Drawing for the job (mm, zero at the part's lowest x, y, z). Coordinates: 2 decimals unless noted, no trailing zeros. Loops run counter-clockwise (first coordinate to the right, second up) from the corner with the lowest first, then second, coordinate; pieces in that order, holes last. Notation, with made-up numbers: (-1, 36) - (8, 36) arc R7 ccw to (8, 46) - close; hole circle Ø2 at (88.5, 88). An arc over 180 degrees is marked (long way). Put each result on its own line as item: value.
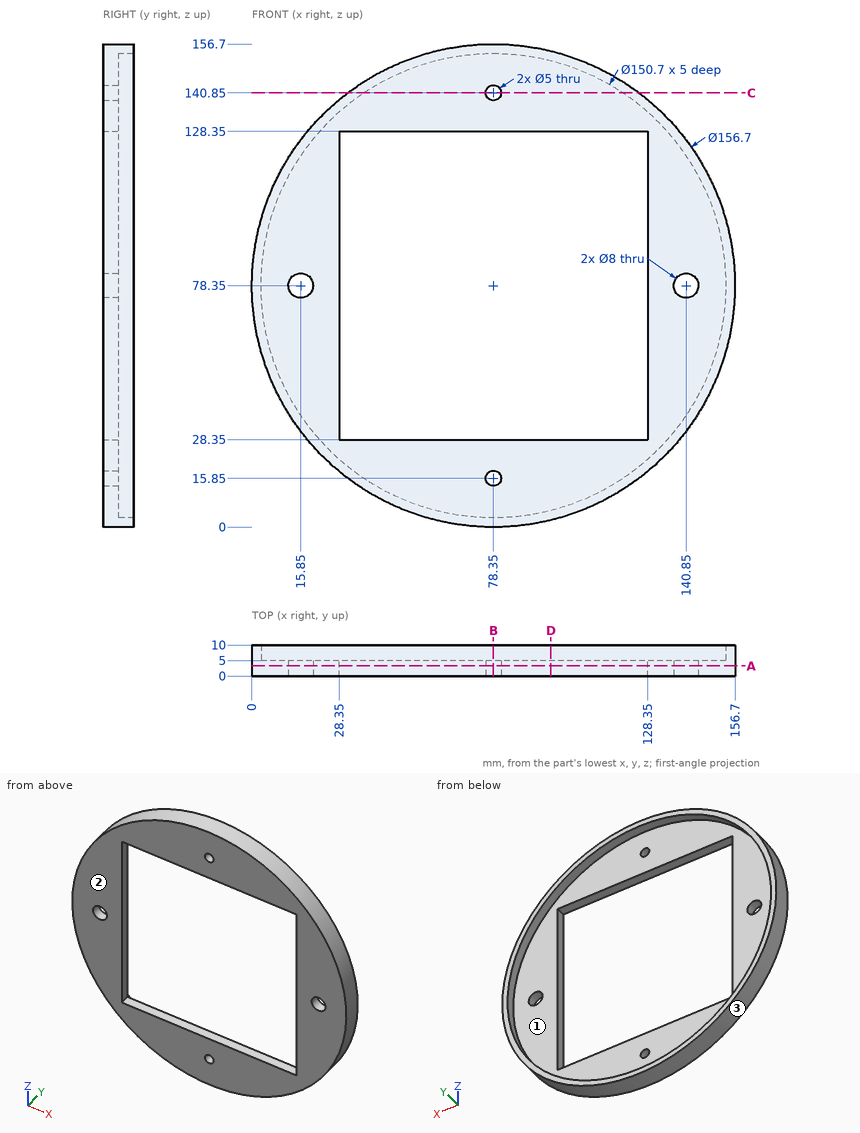
Q1. Slice it at D-D, the plane x = 97. Give the cut face in (y, z), then the cut area to 3 significant figures.
Determined:
outline: (0, 2.25) - (10, 2.25) - (10, 5.34) - (5, 5.34) - (5, 28.35) - (0, 28.35) - close; (0, 128.35) - (5, 128.35) - (5, 151.36) - (10, 151.36) - (10, 154.45) - (0, 154.45) - close
area: 292 mm2
Q2. Slice it at A-A, the plane y = 3.25. Give the cut face in (x, z).
Determined:
outline: circle Ø156.7 at (78.35, 78.35); hole circle Ø8 at (15.85, 78.35); hole (28.35, 28.35) - (128.35, 28.35) - (128.35, 128.35) - (28.35, 128.35) - close; hole circle Ø5 at (78.35, 15.85); hole circle Ø5 at (78.35, 140.85); hole circle Ø8 at (140.85, 78.35)
Q3. Slice it at B-B, the plane x = 78.35. Give the cut face in (y, z), then the cut area to 4 significant figures.
Determined:
outline: (0, 0) - (10, 0) - (10, 3) - (5, 3) - (5, 13.35) - (0, 13.35) - close; (0, 18.35) - (5, 18.35) - (5, 28.35) - (0, 28.35) - close; (0, 128.35) - (5, 128.35) - (5, 138.35) - (0, 138.35) - close; (0, 143.35) - (5, 143.35) - (5, 153.7) - (10, 153.7) - (10, 156.7) - (0, 156.7) - close
area: 263.5 mm2
Q4. Pin check, flat tips, straight feed: pin 1 Ø5.5 at (y, z) = (3.5, 102.5) entering from -X; pin 2 Ø3 at (x, z) = (134, 31) entering from +Y; pin 3 Ø5 at (x, y) = (110.5, 4.5) entering from +Z. Stop position of each tip, or through.
Determined:
pin 1: x = 2.98
pin 2: y = 5
pin 3: z = 150.87
Q5. Slice it at C-C, the plane z = 140.85. Give the cut face in (x, y).
Determined:
outline: (31.1, 0) - (75.85, 0) - (75.85, 5) - (36.26, 5) - (36.26, 10) - (31.1, 10) - close; (80.85, 0) - (125.6, 0) - (125.6, 10) - (120.44, 10) - (120.44, 5) - (80.85, 5) - close
Q6. Wall check: L1, parallel to X at y = 2.25, z = 78.35; L2, parallel to Z at x = 78.5, y = 2.75; L3, parallel to Y at x = 145, z = 55. Give the ranges that are in metal, low to high. Write a range as from..to.
Determined:
L1: 0..11.85, 19.85..28.35, 128.35..136.85, 144.85..156.7
L2: 0..13.35, 18.35..28.35, 128.35..138.35, 143.35..156.7
L3: 0..5
Q7. Mould opens along X. For the marked faces 1, 2 and 3 say: +X half, -X half, draft (parallel to the pull), parting line (faces both ways), or undercut.
Determined:
face 1: undercut
face 2: draft
face 3: parting line
